Design review of the part built by this model. Coordinates are the model's own, in mm. A direction names the side the tool comes from. Coordinates: 2 decimals unless noted, no trailing zeros. Order: outer loops, then holes, each group sorted by start corner. A loop starts at its lowest first (then second) coordinate and runs counter-clockwise, first axis right, second up. Notation, with made-up numbers: (89, 31) -> (134, 31) arc R31 cw to (134, 64) -> close; hole circle Ø5 at (24.25, 89.5). An arc over 180 degrees is marked (long way). Use a Markdown table: item, result. Add a question column.
Q1. The part is to be moulded in two halves that separate along X. For faces 1 (the face through (37.1, 0, 52)), 2 (the face through (-1, -20.75, 52)), 3 (the face through (-18, -15, 2)), say which applies: pulls with the +X half, pulls with the -X half, needs draft (parallel to the pull), parting line crosses it, or undercut.
Q2. Add section D-D (x = 23.6). State the section outline as (y, z) points, then the cut area to 3 significant figures.
Q3. Add section B-B (x = -31). State the section outline as (y, z) points, then the cut area to 3 significant figures.
Q4. Insertion check: pin 1 (21 mm diameter, centred on x = 15.5, y = -2, fed in from +Z); pin 2 (2 mm diameter, centred on x = -4.5, y = -5, fed in from -Z); pin 3 (0.8 mm diameter, centred on y = -16.5, z = 5.5, fed in from -X); pin 4 (4 mm diameter, centred on x = 11, y = 10.5, fed in from -Z). Each pin has a flat end and moves straight along its axis. Give the tip position at first contact, or say it passes through.
Q5. Machinability: for faces 4 (the face through (-34, -15, 2)), 5 (the face through (25, 0, 18)), 6 (the face through (39, 0, 41)), which of the approach directions +Z, -Z, +X, -X, +Y, -Y give a long, thin tool a straight path to every point of the face, cutting with its end or side? Answer none if there is none.
Q6. Wall thickness on probe 1 along Z at (x, y) = (-5, -22.5); probe 2 along Y at (x, z) = (23.6, 1.3); probe 3 along Y at (x, z) = (-12, 12.5): over which ranges is each line inside the solid? List them lowest first.
Q7. Add section A-A (y = 0). Count the separate pieces of the cut face and the enclosed holes in it, then the cut area to 3 significant figures.
Q8. Add section C-C (z = 40). State the section outline as (x, y) points, then the cut area to 3 significant figures.
from build123d import *

# Parameters (mm, degrees)
ESQUISSE1_W              = 82.2
ESQUISSE1_H              = 49.5
BOSS_EXTRU_1_DEPTH       = 3
ESQUISSE2_W              = 82.2
ESQUISSE2_H              = 49.5
ESQUISSE2_W_2            = 74.2
ESQUISSE2_H_2            = 41.5
BOSS_EXTRU_2_DEPTH       = 50
ESQUISSE4_W              = 2
ESQUISSE4_H              = 41.5
ENL_V_MAT_EXTRU_3_DEPTH  = 16
ENL_V_MAT_EXTRU_4_DEPTH  = 80.2
ESQUISSE6_W              = 46
ESQUISSE6_H              = 41.5
ENL_V_MAT_EXTRU_5_DEPTH  = 10
ESQUISSE7_W              = 5
ESQUISSE7_H              = 9
BOSS_EXTRU_3_DEPTH       = 20
CHANFREIN1_SIZE          = 5
CHANFREIN2_SIZE          = 2
CHANFREIN3_SIZE          = 2
ESQUISSE8_R              = 6.75
ENL_V_MAT_EXTRU_6_DEPTH  = 5
ESQUISSE10_W             = 26.9
ESQUISSE10_H             = 17
BOSS_EXTRU_4_DEPTH       = 4.5
ESQUISSE9_W              = 33
ESQUISSE9_H              = 12.2
ENL_V_MAT_EXTRU_8_DEPTH  = 5
ESQUISSE11_W             = 2.2
ESQUISSE11_H             = 12.2
ENL_V_MAT_EXTRU_9_DEPTH  = 7
ESQUISSE12_W             = 18
ESQUISSE12_H             = 11
ENL_V_MAT_EXTRU_10_DEPTH = 2
ESQUISSE13_W             = 4.5
ESQUISSE13_H             = 11
ENL_V_MAT_EXTRU_11_DEPTH = 3
ESQUISSE14_W             = 4
ESQUISSE14_H             = 11
BOSS_EXTRU_5_DEPTH       = 3
ESQUISSE15_W             = 4
ESQUISSE15_H             = 11
ENL_V_MAT_EXTRU_12_DEPTH = 3
ESQUISSE16_W             = 7
ESQUISSE16_H             = 1.5
BOSS_EXTRU_6_DEPTH       = 3
CHANFREIN4_SIZE          = 3
ESQUISSE18_W             = 0.2
ESQUISSE18_H             = 1.5
ESQUISSE18_W_2           = 4.5
BOSS_EXTRU_8_DEPTH       = 3
ESQUISSE19_W             = 3
ESQUISSE19_H             = 1.25
BOSS_EXTRU_9_DEPTH       = 3
ESQUISSE20_W             = 1.7
ESQUISSE20_H             = 2
BOSS_EXTRU_10_DEPTH      = 11
CHANFREIN10_SIZE         = 3.247037966
CHANFREIN10_SIZE_2       = 5
CHANFREIN11_SIZE         = 2
ESQUISSE21_W             = 8
ESQUISSE21_H             = 12
ENL_V_MAT_EXTRU_13_DEPTH = 10


with BuildPart() as part:
    # Esquisse1 → Boss.-Extru.1 (new body)
    with BuildSketch(Plane.XY):
        Rectangle(ESQUISSE1_W, ESQUISSE1_H)
    extrude(amount=BOSS_EXTRU_1_DEPTH)

    # Esquisse2 → Boss.-Extru.2 (add)
    with BuildSketch(Plane.XY.offset(3)):
        Rectangle(ESQUISSE2_W, ESQUISSE2_H)
        Rectangle(ESQUISSE2_W_2, ESQUISSE2_H_2, mode=Mode.SUBTRACT)
    extrude(amount=BOSS_EXTRU_2_DEPTH)

    # Esquisse4 → Enlèv. mat.-Extru.3 (cut)
    with BuildSketch(Plane(origin=(-37.1, 0, 0), x_dir=(0, 0, -1), z_dir=(1, 0, 0))):
        with Locations((-52, 0)):
            Rectangle(ESQUISSE4_W, ESQUISSE4_H)
    extrude(amount=-ENL_V_MAT_EXTRU_3_DEPTH, mode=Mode.SUBTRACT)

    # Esquisse5 → Enlèv. mat.-Extru.4 (cut)
    with BuildSketch(Plane.ZY.offset(41.1)):
        Polygon((51, 22.75), (49, 22.75), (49, -22.75), (51, -22.75), (51, -20.75), (51, 20.75), align=None)
    extrude(amount=-ENL_V_MAT_EXTRU_4_DEPTH, mode=Mode.SUBTRACT)

    # Esquisse6 → Enlèv. mat.-Extru.5 (cut)
    with BuildSketch(Plane(origin=(-37.1, 0, 0), x_dir=(0, 0, -1), z_dir=(1, 0, 0))):
        with Locations((-26, 0)):
            Rectangle(ESQUISSE6_W, ESQUISSE6_H)
    extrude(amount=-ENL_V_MAT_EXTRU_5_DEPTH, mode=Mode.SUBTRACT)

    # Esquisse7 → Boss.-Extru.3 (add)
    with BuildSketch(Plane.ZY.offset(-37.1)):
        with Locations((15.5, 0)):
            Rectangle(ESQUISSE7_W, ESQUISSE7_H)
    extrude(amount=BOSS_EXTRU_3_DEPTH)

    # Chanfrein1
    chanfrein1_edges = [part.edges().sort_by_distance(p)[0] for p in [
        (37.1, 0, 18),
    ]]
    chamfer(chanfrein1_edges, length=CHANFREIN1_SIZE)

    # Chanfrein2
    chanfrein2_edges = [part.edges().sort_by_distance(p)[0] for p in [
        (37.1, 0, 13),
    ]]
    chamfer(chanfrein2_edges, length=CHANFREIN2_SIZE)

    # Chanfrein3
    chanfrein3_edges = [part.edges().sort_by_distance(p)[0] for p in [
        (37.1, -4.5, 17),
        (37.1, 4.5, 17),
    ]]
    chamfer(chanfrein3_edges, length=CHANFREIN3_SIZE)

    # Esquisse8 → Enlèv. mat.-Extru.6 (cut)
    with BuildSketch(Plane(origin=(0, 0, 0), x_dir=(-1, 0, 0), z_dir=(0, 0, -1))):
        with Locations((-23.6, 0)):
            Circle(ESQUISSE8_R)
    extrude(amount=-ENL_V_MAT_EXTRU_6_DEPTH, mode=Mode.SUBTRACT)

    # Esquisse10 → Boss.-Extru.4 (add)
    with BuildSketch(Plane.XY.offset(3)):
        with Locations((-7.45, 0)):
            Rectangle(ESQUISSE10_W, ESQUISSE10_H)
    extrude(amount=BOSS_EXTRU_4_DEPTH)

    # Esquisse9 → Enlèv. mat.-Extru.8 (cut)
    with BuildSketch(Plane(origin=(0, 0, 0), x_dir=(-1, 0, 0), z_dir=(0, 0, -1))):
        with Locations((12.9, 0)):
            Rectangle(ESQUISSE9_W, ESQUISSE9_H)
    extrude(amount=-ENL_V_MAT_EXTRU_8_DEPTH, mode=Mode.SUBTRACT)

    # Esquisse11 → Enlèv. mat.-Extru.9 (cut)
    with BuildSketch(Plane(origin=(-29.4, 0, 0), x_dir=(0, 0, -1), z_dir=(1, 0, 0))):
        with Locations((-1.9, 0)):
            Rectangle(ESQUISSE11_W, ESQUISSE11_H)
    extrude(amount=-ENL_V_MAT_EXTRU_9_DEPTH, mode=Mode.SUBTRACT)

    # Esquisse12 → Enlèv. mat.-Extru.10 (cut)
    with BuildSketch(Plane(origin=(0, 0, 0), x_dir=(-1, 0, 0), z_dir=(0, 0, -1))):
        with Locations((26.1, -15.25)):
            Rectangle(ESQUISSE12_W, ESQUISSE12_H)
    extrude(amount=-ENL_V_MAT_EXTRU_10_DEPTH, mode=Mode.SUBTRACT)

    # Esquisse13 → Enlèv. mat.-Extru.11 (cut)
    with BuildSketch(Plane(origin=(0, 0, 2), x_dir=(-1, 0, 0), z_dir=(0, 0, -1))):
        with Locations((21.85, -15.25)):
            Rectangle(ESQUISSE13_W, ESQUISSE13_H)
        with Locations((30.35, -15.25)):
            Rectangle(ESQUISSE13_W, ESQUISSE13_H)
    extrude(amount=-ENL_V_MAT_EXTRU_11_DEPTH, mode=Mode.SUBTRACT)

    # Esquisse14 → Boss.-Extru.5 (add)
    with BuildSketch(Plane.XY.offset(3)):
        with Locations((-26.1, -15.25)):
            Rectangle(ESQUISSE14_W, ESQUISSE14_H)
    extrude(amount=BOSS_EXTRU_5_DEPTH)

    # Esquisse15 → Enlèv. mat.-Extru.12 (cut)
    with BuildSketch(Plane(origin=(0, 0, 2), x_dir=(-1, 0, 0), z_dir=(0, 0, -1))):
        with Locations((26.1, -15.25)):
            Rectangle(ESQUISSE15_W, ESQUISSE15_H)
    extrude(amount=-ENL_V_MAT_EXTRU_12_DEPTH, mode=Mode.SUBTRACT)

    # Esquisse16 → Boss.-Extru.6 (add)
    with BuildSketch(Plane.XY.offset(3)):
        with Locations((-24.6, -9)):
            Rectangle(ESQUISSE16_W, ESQUISSE16_H)
    extrude(amount=BOSS_EXTRU_6_DEPTH)

    # Chanfrein4
    chanfrein4_edges = [part.edges().sort_by_distance(p)[0] for p in [
        (6, 0, 3),
    ]]
    chamfer(chanfrein4_edges, length=CHANFREIN4_SIZE)

    # Esquisse18 → Boss.-Extru.8 (add)
    with BuildSketch(Plane.XY.offset(3)):
        with Locations((-21, -9)):
            Rectangle(ESQUISSE18_W, ESQUISSE18_H)
        with Locations((-30.35, -9)):
            Rectangle(ESQUISSE18_W_2, ESQUISSE18_H)
    extrude(amount=BOSS_EXTRU_8_DEPTH)

    # Esquisse19 → Boss.-Extru.9 (add)
    with BuildSketch(Plane(origin=(-20.9, 0, 0), x_dir=(0, 0, -1), z_dir=(1, 0, 0))):
        with Locations((-4.5, -9.125)):
            Rectangle(ESQUISSE19_W, ESQUISSE19_H)
    extrude(amount=BOSS_EXTRU_9_DEPTH)

    # Esquisse20 → Boss.-Extru.10 (add)
    with BuildSketch(Plane(origin=(0, -9.75, 0), x_dir=(-1, 0, 0), z_dir=(0, -1, 0))):
        Polygon((17.9, -6), (24.1, -6), (24.1, -5), (19.6, -5), (17.9, -5), align=None)
        with Locations((18.75, -4)):
            Rectangle(ESQUISSE20_W, ESQUISSE20_H)
    extrude(amount=BOSS_EXTRU_10_DEPTH)

    # Chanfrein10
    # the kernel refuses this chamfer: 5, 3.247037966 mm, written as the material it adds along each edge
    with BuildSketch(Plane(origin=(-17.9, 4.422205001, 3), x_dir=(-0.04991856572298826, 0, 0.9987532912567346), z_dir=(0, -1, 0))) as chanfrein10_piece_1_section:
        Polygon((CHANFREIN10_SIZE * 0.998753291253, -CHANFREIN10_SIZE * 0.0499185657228), (-CHANFREIN10_SIZE_2 * 0.049918565723, -CHANFREIN10_SIZE_2 * 0.998753291257), (0, 0), align=None)
    chanfrein10_piece_1 = extrude(amount=25.172205001, mode=Mode.PRIVATE)
    chanfrein10_piece_1 = split(chanfrein10_piece_1, bisect_by=Plane(origin=(-17.932311405, -8.5, 6.135567439), z_dir=(0, 1, 0)), keep=Keep.TOP, mode=Mode.PRIVATE)
    chanfrein10_piece_1 = split(chanfrein10_piece_1, bisect_by=Plane(origin=(-17.932311405, -2.038897499, 6), z_dir=(0, 0, 1)), keep=Keep.TOP, mode=Mode.PRIVATE)
    add(chanfrein10_piece_1)
    with BuildSketch(Plane(origin=(-17.9, -8.5, 3), x_dir=(-0.04991856572298826, 0, 0.9987532912567346), z_dir=(0, -1, 0))) as chanfrein10_piece_2_section:
        Polygon((CHANFREIN10_SIZE * 0.998753291253, -CHANFREIN10_SIZE * 0.0499185657228), (-CHANFREIN10_SIZE_2 * 0.049918565723, -CHANFREIN10_SIZE_2 * 0.998753291257), (0, 0), align=None)
    chanfrein10_piece_2 = extrude(amount=12.25, mode=Mode.PRIVATE)
    chanfrein10_piece_2 = split(chanfrein10_piece_2, bisect_by=Plane(origin=(-16.206622299, -14.625, 6), z_dir=(0, 0, -1)), keep=Keep.TOP, mode=Mode.PRIVATE)
    add(chanfrein10_piece_2)

    # Chanfrein11
    chanfrein11_edges = [part.edges().sort_by_distance(p)[0] for p in [
        (-20.9, -8.25, 4.5),
    ]]
    chamfer(chanfrein11_edges, length=CHANFREIN11_SIZE)

    # Esquisse21 → Enlèv. mat.-Extru.13 (cut)
    with BuildSketch(Plane(origin=(41.1, 0, 0), x_dir=(0, 0, -1), z_dir=(1, 0, 0))):
        with Locations((-45, 0)):
            Rectangle(ESQUISSE21_W, ESQUISSE21_H)
    extrude(amount=-ENL_V_MAT_EXTRU_13_DEPTH, mode=Mode.SUBTRACT)


solid = part.part
Established:
| question | item | result |
|---|---|---|
| 1 | face 1 | pulls with the -X half |
| 1 | face 2 | needs draft |
| 1 | face 3 | undercut |
| 2 | outline | (-24.75, 0) -> (-6.75, 0) -> (-6.75, 3) -> (-20.75, 3) -> (-20.75, 49) -> (-22.75, 49) -> (-22.75, 51) -> (-20.75, 51) -> (-20.75, 53) -> (-24.75, 53) -> close; (-4.5, 13) -> (4.5, 13) -> (4.5, 18) -> (-4.5, 18) -> close; (6.75, 0) -> (24.75, 0) -> (24.75, 53) -> (20.75, 53) -> (20.75, 51) -> (22.75, 51) -> (22.75, 49) -> (20.75, 49) -> (20.75, 3) -> (6.75, 3) -> close |
| 2 | area | 545 mm^2 |
| 3 | outline | (-24.75, 0) -> (-20.75, 0) -> (-20.75, 49) -> (-22.75, 49) -> (-22.75, 51) -> (-20.75, 51) -> (-20.75, 53) -> (-24.75, 53) -> close; (-9.75, 0) -> (24.75, 0) -> (24.75, 53) -> (20.75, 53) -> (20.75, 51) -> (22.75, 51) -> (22.75, 49) -> (20.75, 49) -> (20.75, 3) -> (6.1, 3) -> (6.1, 0.8) -> (-6.1, 0.8) -> (-6.1, 3) -> (-8.25, 3) -> (-8.25, 6) -> (-9.75, 6) -> close |
| 3 | area | 485 mm^2 |
| 4 | pin 1 | z = 18 |
| 4 | pin 2 | z = 5 |
| 4 | pin 3 | x = -28.1 |
| 4 | pin 4 | z = 0 |
| 5 | face 4 | -Z |
| 5 | face 5 | +Z, -X |
| 5 | face 6 | +X, -X |
| 6 | probe 1 | 0 to 49, 51 to 53 |
| 6 | probe 2 | -24.75 to -6.75, 6.75 to 24.75 |
| 6 | probe 3 | -24.75 to -20.75, 20.75 to 24.75 |
| 7 | separate pieces | 4 |
| 7 | enclosed holes | 0 |
| 7 | area | 447 mm^2 |
| 8 | outline | (-41.1, -24.75) -> (41.1, -24.75) -> (41.1, 24.75) -> (-41.1, 24.75) -> (-41.1, 20.75) -> (37.1, 20.75) -> (37.1, -20.75) -> (-41.1, -20.75) -> close |
| 8 | area | 824 mm^2 |
